```python
from build123d import *

# Parameters (mm, degrees)
SKETCH059_R     = 12.5
PAD030_DEPTH    = 8
SKETCH060_R     = 3.5
POCKET029_DEPTH = 6.5
FILLET003_R     = 1
SKETCH061_R     = 2
POCKET030_DEPTH = 10


with BuildPart() as part:
    # Sketch059 → Pad030 (new body)
    with BuildSketch(Plane.XY):
        Circle(SKETCH059_R)
    extrude(amount=PAD030_DEPTH)

    # Sketch060 (on Face2 of Pad030) → Pocket029 (cut)
    with BuildSketch(Plane(origin=(0, 0, 0), x_dir=(1, 0, 0), z_dir=(0, 0, -1))):
        Circle(SKETCH060_R)
    extrude(amount=-POCKET029_DEPTH, mode=Mode.SUBTRACT)

    # Fillet003
    fillet003_edges = [part.edges().sort_by_distance(p)[0] for p in [
        (-12.5, 0, 8),
    ]]
    fillet(fillet003_edges, radius=FILLET003_R)

    # Sketch061 (on DatumPlane) → Pocket030 (cut)
    with BuildSketch(Plane(origin=(0, 12.5, 3.5), x_dir=(-1, 0, 0), z_dir=(0, 1, 0))):
        Circle(SKETCH061_R)
    extrude(amount=-POCKET030_DEPTH, mode=Mode.SUBTRACT)


with BuildPart() as part_1:
    # Body015 placement: moved
    add(part.part.moved(Location((94.5, 67.5, 2.5))))


solid = part_1.part
```
For this review, take the finished solid that the model builds, in its own axes (mm). A direction names the side the tool comes from. Round coordinates to 2 decimals unless told otherwise and drop trailing zeros. Write each loop counter-clockwise with the first axis right and the second up, starting at its lowest first coordinate (ties: lowest second). Pieces come first, ordered by that corner, then holes. Notation, with made-up numbers: (88.5, -1) -> (95.5, -1) arc R24 ccw to (95.5, 10) -> close; hole circle Ø4 at (89.5, 43.25). An arc over 180 degrees is marked (long way). Use one line per item in the form item = value.
1) Take a section at D-D, the plane z = 6. Write out the cut boundary in (x, y), and give its area (3 significant figures).
Found:
outline = (92.5, 70.37) -> (92.5, 79.84) arc R12.5 ccw (long way) to (96.5, 79.84) -> (96.5, 70.37) arc R3.5 cw (long way) to start
area = 416 mm2
2) To check wall thickness, follow L1, parallel to Z at x = 94.5, y = 74; L2, parallel to Z at x = 92.5, y = 65.25; L3, parallel to Y at x = 94.5, z = 7.25. State the ranges of each line that lie inside material, in increasing order. Write a range as from..to.
Found:
L1 = 2.5..4, 8..10.5
L2 = 9..10.5
L3 = 55..64
3) Take a section at A-A, the plane x = 94.5. Write out the cut boundary in (y, z), and give its area (3 significant figures).
Found:
outline = (55, 2.5) -> (64, 2.5) -> (64, 9) -> (71, 9) -> (71, 8) -> (80, 8) -> (80, 9.5) arc R1 ccw to (79, 10.5) -> (56, 10.5) arc R1 ccw to (55, 9.5) -> close; (71, 2.5) -> (80, 2.5) -> (80, 4) -> (71, 4) -> close
area = 118 mm2
4) Clearance check with flat-ended pins moving along their axes: pin 1 (5.5 mm diameter, centred on x = 94.5, y = 67.5, fed in from -Z); pin 2 (2 mm diameter, centred on y = 65, z = 7.5, fed in from +X); pin 3 (3 mm diameter, centred on x = 85, y = 77, fed in from +Z). State where each tip first meets the part, or that it passes through.
Found:
pin_1 = 9
pin_2 = 106.91
pin_3 = 10.4
5) Mouldability with a two-part tool opening along X and no side actions: class faces 3 (the flat face through (97.1, 64.9, 2.5)), 4 (the cylindrical face through (93.577, 75.254, 4.226)), 5 (the cylindrical face through (100.27, 56.41, 5.95)) as +X half, -X half, draft (parallel to the pull), parting line (faces both ways), or undercut.
Found:
face_3 = draft
face_4 = undercut
face_5 = parting line
6) Take a section at C-C, the plane z = 8.5. Write out the cut boundary in (x, y), and give its area (3 significant figures).
Found:
outline = circle Ø25 at (94.5, 67.5); hole circle Ø7 at (94.5, 67.5)
area = 452 mm2
7) Tool access review of faces 1 (the flat face through (94, 68, 10.5)), 2 (the cylindrical face through (94.04, 64.03, 5.7)): name each direction out of +Z, -Z, +X, -X, +Y, -Y from which nothing blocks a thin tool from reaching the whole face with its end or side.
Found:
face_1 = +Z, +X, -X, +Y, -Y
face_2 = -Z
8) Take a section at B-B, the plane y = 67.5. Write out the cut boundary in (x, z).
Found:
outline = (82, 2.5) -> (91, 2.5) -> (91, 9) -> (98, 9) -> (98, 2.5) -> (107, 2.5) -> (107, 9.5) arc R1 ccw to (106, 10.5) -> (83, 10.5) arc R1 ccw to (82, 9.5) -> close
